Part model, mm, in its own coordinate system. Face numbers are marked on the shaded views. Round coordinates to 2 decimals unless told otherwise and drop trailing zeros. Loops run counter-clockwise (first coordinate to the right, second up) from the corner with the lowest first, then second, coordinate; pieces in that order, holes last. Notation, with made-up numbers: M 75.25,14.25 L 110.25,14.25 A27 ccw 110.25,39.25 Z; hole C -19,27 d2. An arc over 180 degrees is marked long. Put each result on its own line as item: value. Start each with the question number.
```python
from build123d import *

# Parameters (mm, degrees)
SKETCH1_R                = 10
BOSS_EXTRUDE1_DEPTH      = 12.5
BOSS_EXTRUDE1_DEPTH_BACK = 12.5
SKETCH2_R                = 10
BOSS_EXTRUDE2_DEPTH      = 17.5


with BuildPart() as part:
    # Sketch1 → Boss-Extrude1 (new body, two sides)
    with BuildSketch(Plane.XY) as boss_extrude1_sk:
        with BuildLine():
            ThreePointArc((9.980766544, 59.380081301), (0, 70), (-9.980766544, 59.380081301))
            ThreePointArc((-9.980766544, 59.380081301), (-10.573802909, 1.597827145), (-19.486258491, -55.496031746))
            ThreePointArc((-19.486258491, -55.496031746), (0, -80), (19.486258491, -55.496031746))
            ThreePointArc((19.486258491, -55.496031746), (10.573802909, 1.597827145), (9.980766544, 59.380081301))
        make_face()
        with Locations((0, -60)):
            Circle(SKETCH1_R, mode=Mode.SUBTRACT)
    extrude(amount=BOSS_EXTRUDE1_DEPTH)
    extrude(boss_extrude1_sk.sketch, amount=-BOSS_EXTRUDE1_DEPTH_BACK)

    # Sketch2 → Boss-Extrude2 (add)
    with BuildSketch(Plane.XY.offset(12.5)):
        with Locations((0, 60)):
            Circle(SKETCH2_R)
    boss_extrude2 = extrude(amount=BOSS_EXTRUDE2_DEPTH)

    # Mirror1: Boss-Extrude2 across plane
    add(boss_extrude2.mirror(Plane.XY))


solid = part.part
```
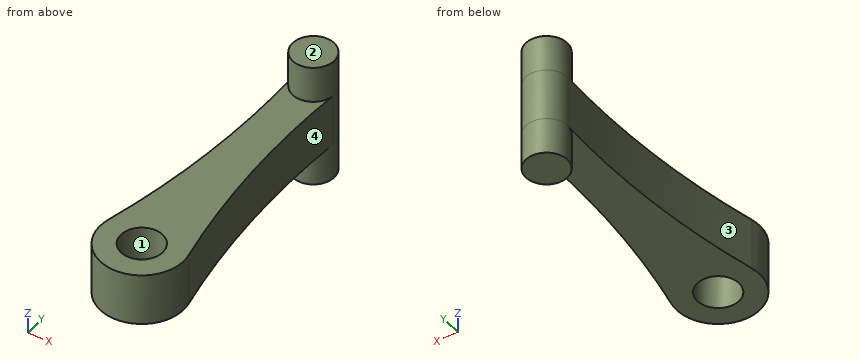
1. Drop flat-ended pins along their axis: pin 1 (1.5 mm diameter, centred on y = -49, z = -8.5, fed in from -X); pin 2 (5 mm diameter, centred on y = 25.5, z = -13.5, fed in from +X); pin 3 (3 mm diameter, centred on x = 4.5, z = -23.5, fed in from +Y). Give the stop position or say it passes through.
2. Cut at A-A, the plane y = -60. Give the cut face in (x, z).
3. Cut at D-D, the plane z = -23. Give the cut face in (x, y), and give its area (3 significant figures).
4. Cut at C-C, the plane z = 6.5. Give the cut face in (x, y).
5. Mould opens along X. For the marked faces 1, 2, 3 and 4 say: released by +X, released by -X, zero draft, split by the parting line, or undercut.
6. Wall check: L1, parallel to Z at x = -16, y = -47; L2, parallel to Y at x = 6.5, z = 5; L3, parallel to Y at x = -1.5, z = 11. Give the ranges that are in metal, low to high.
7. Cut at B-B, the plane x = 0. Give the cut face in (y, z).
Results list:
1. pin 1: stops at x = -18.2
1. pin 2: stops at x = 9.37
1. pin 3: stops at y = 69.54
2. outline: M -20,-12.5 L -10,-12.5 L -10,12.5 L -20,12.5 Z; M 10,-12.5 L 20,-12.5 L 20,12.5 L 10,12.5 Z
3. outline: C 0,60 d20
3. area: 314 mm^2
4. outline: M -19.49,-55.5 A20 ccw long 19.49,-55.5 A400 cw 9.98,59.38 A10 ccw long -9.98,59.38 A400 cw Z; hole C 0,-60 d20
5. face 1: undercut
5. face 2: zero draft
5. face 3: released by -X
5. face 4: released by +X
6. L1: z = -12.5 to 12.5
6. L2: y = -78.91 to -67.6, -52.4 to 67.6
6. L3: y = -79.94 to -69.89, -50.11 to 69.89
7. outline: M -80,-12.5 L -70,-12.5 L -70,12.5 L -80,12.5 Z; M -50,-12.5 L 50,-12.5 L 50,-30 L 70,-30 L 70,30 L 50,30 L 50,12.5 L -50,12.5 Z
